Autodesk Inventor part; units mm, degrees
ref_plane "YZ Plane" through (0, 0, 0) normal (1, 0, 0) x (0, 1, 0)
ref_plane "XZ Plane" through (0, 0, 0) normal (0, 1, 0) x (-1, 0, 0)
ref_plane "XY Plane" through (0, 0, 0) normal (0, 0, 1) x (1, 0, 0)
sketch "Sketch1" plane through (0, 0, 0) normal (0, 1, 0) x (-1, 0, 0)
  line L0 (15, 20) -> (-15, 20)
  line L1 (-15, 20) -> (-15, -20)
  line L2 (-15, -20) -> (15, -20)
  line L3 (15, -20) -> (15, 20)
  line L4 (15, 20) -> (-15, -20) construction
  line L5 (-15, 20) -> (15, -20) construction
  line L6 (21, 0) -> (-21, 0) construction
  line L7 (0, -28) -> (0, 28) construction
  line L8 (6, 0) -> (0, 0) construction
  line L9 (6, 3.4) -> (0, 3.4)
  line L10 (0, -3.4) -> (6, -3.4)
  arc A0 (6, -3.4) -> (6, 3.4) centre (6, 0) ccw
  arc A1 (0, 3.4) -> (0, -3.4) centre (0, 0) ccw
  line L11 (-15, 12.5) -> (15, 12.5)
  line L12 (-15, -12.5) -> (15, -12.5)
  point P0 (0, 0)
  point P1 (3, 0)
  point P2 (3, 0)
  point P3 (15, -12.5)
  dimension "d0" = 40
  dimension "d1" = 30
  dimension "d2" = 6
  dimension "d3" = 6.8
  dimension "d19" = 3
  dimension "d35" = 25
extrude "Extrusion1" add sketch "Sketch1" against normal blind 28 contours L3 L11 L1 L0 | L3 L12 L1 L11 | L3 L2 L1 L12 | A0 L10 A1 L9
extrude "Extrusion2" cut sketch "Sketch1" against normal blind 8
sketch "Sketch3" plane through (0, -28, 0) normal (0, -1, 0) x (1, 0, 0)
  circle A0 centre (0, 0) radius 7.5
  dimension "d29" = 15
extrude "Extrusion5" cut sketch "Sketch3" against normal blind 15
extrude "Extrusion6" cut sketch "Sketch1" against normal blind 23 contours L3 L11 L1 L0 | L3 L2 L1 L12
hole "Hole1" at (-3, 0, 0) direction (0, -1, 0) diameter 4.917 depth 13 countersink diameter 6 countersink angle 90
fillet "Fillet1" radius 5 4 edges at (-15, -25.5, 20) (-15, -25.5, -20) (15, -25.5, -20) (15, -25.5, 20)
chamfer "Chamfer1" distance 0.5 angle 45 13 edges at (0, -28, 20) (-13.5355, -28, 18.5355) (-15, -28, 0) (-13.5355, -28, -18.5355) (0, -28, -20) (13.5355, -28, -18.5355) (15, -28, 0) (13.5355, -28, 18.5355) (-7.5, -28, 0) (-15, -15.5, 12.5) (-15, -15.5, -12.5) (15, -15.5, -12.5) (15, -15.5, 12.5)
equation "\"d4\" = slotTabH + sheetT"
equation "\"d6\" = slotTabH"
equation "\"slotTabH\" = 8"
equation "\"sheetT\" = 20"
equation "\"totalHeight\" = slotTabH + sheetT"
properties part number "TCSM1-X-003" material "Steel"
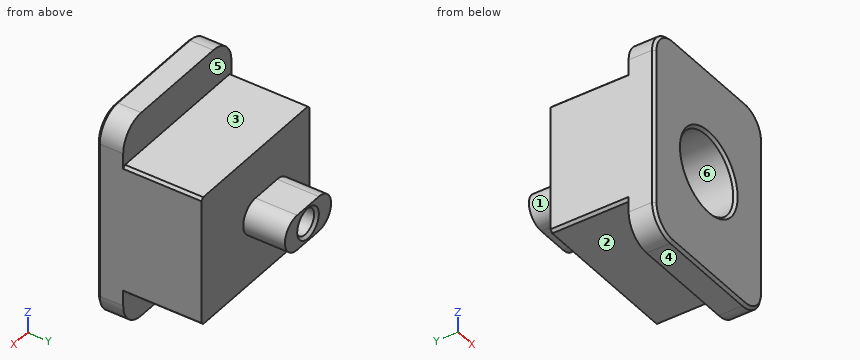
The listing builds one solid part. Answer for the finished solid, in the listing's coordinates (mm). Face numbers are marked on the shaded views. A direction names the side the tool comes from. Coordinates: 2 decimals unless noted, no trailing zeros. Loops run counter-clockwise (first coordinate to the right, second up) from the corner with the lowest first, then second, coordinate; pieces in that order, holes last. Notation, with made-up numbers: (-10.75, -19.75) -> (45.25, -19.75) arc R14 ccw to (45.25, -10.75) -> close; hole circle Ø1 at (18, 85.5). An arc over 180 degrees is marked (long way). Use one line per item in the form item = value. Start each with the question number.
Item 1: The part is cut by section B-B on y = -12.5. Determine the outline of the cut face in (x, z), then the cut area to 3 significant figures.
Item 2: The part is cut by section A-A on z = 0. Determine the outline of the cut face in (x, y).
Item 3: Flat-ended cylindrical pins translate along their axes: pin 1 Ø1.8 at (x, y) = (-2.5, -3.5) entering from -Z; pin 2 Ø6.5 at (x, z) = (2.5, -14.5) entering from +Y; pin 3 Ø9 at (x, z) = (0, 0) entering from -Y; pin 4 Ø4 at (x, z) = (-3, 0) entering from +Y. Find the tip coordinate at first contact, or state that the pin passes through.
Item 4: A tool of negligible diameter and unlimited length cuts with its end or side. For the marked faces 1, 2 and 3, from which of +Z, -Z, +X, -X, +Y, -Y can it reach the whole face along a straight path? Write none if from no direction.
Item 5: Consider L1, parallel to Z at x = -3, y = -6.5; L2, parallel to X at y = -4, z = 0; L3, parallel to Z at x = 0, y = -19. Determine where each line is inside the solid, lowest interval first. Write a range as [from, to].
Item 6: The mould has two halves that part along Z. Classify the marked faces 4, 5 and 6: released by +Z, released by -Z, zero draft, split by the parting line, or undercut.
Item 7: The part is cut by section D-D on y = -6.75. Determine the outline of the cut face in (x, z).
Item 8: The part is cut by section C-C on z = -13. Determine the outline of the cut face in (x, y), then the cut area to 3 significant figures.
Answer key:
q1.outline = (-15, -12) -> (-14.5, -12.5) -> (14.5, -12.5) -> (15, -12) -> (15, 12) -> (14.5, 12.5) -> (-14.5, 12.5) -> (-15, 12) -> close; hole circle Ø4.92 at (-3, 0)
q1.area = 731 mm2
q2.outline = (-15, -27.5) -> (-14.5, -28) -> (-8, -28) -> (-7.5, -27.5) -> (-7.5, -13) -> (-5.46, -13) -> (-5.46, -0.54) -> (-6, 0) -> (-9.4, 0) -> (-9.4, -8) -> (-15, -8) -> close; (-0.54, -13) -> (7.5, -13) -> (7.5, -27.5) -> (8, -28) -> (14.5, -28) -> (15, -27.5) -> (15, -8) -> (3.4, -8) -> (3.4, 0) -> (0, 0) -> (-0.54, -0.54) -> close
q3.pin_1 = -3.4
q3.pin_2 = -8
q3.pin_3 = -13
q3.pin_4 = through
q4.face_1 = -X, +Y
q4.face_2 = -Z, +X, -X, +Y
q4.face_3 = +Z, +X, -X, +Y
q5.L1 = [-3.4, -2.46], [2.46, 3.4]
q5.L2 = [-9.4, -5.46], [-0.54, 3.4]
q5.L3 = [-12.5, -7.5], [7.5, 12.5]
q6.face_4 = released by -Z
q6.face_5 = zero draft
q6.face_6 = undercut
q7.outline = (-6, -3.4) -> (0, -3.4) arc R3.4 ccw to (0, 3.4) -> (-6, 3.4) arc R3.4 ccw to start; hole circle Ø4.92 at (-3, 0)
q8.outline = (-15, -27.5) -> (-14.5, -28) -> (14.5, -28) -> (15, -27.5) -> (15, -23) -> (-15, -23) -> close
q8.area = 150 mm2
